The listing builds one solid part. Answer for the finished solid, in the listing's coordinates (mm). Face numbers are marked on the shaded views. A direction names the side the tool comes from. Coordinates: 2 decimals unless noted, no trailing zeros. Write each loop counter-clockwise with the first axis right and the second up, starting at its lowest first coordinate (ties: lowest second). Pieces come first, ordered by that corner, then holes.
from build123d import *

# Parameters (mm, degrees)
BASE_FLANGE1_DEPTH             = 120.65
BASE_FLANGE1_DEPTH_BACK        = 120.65
SKETCH2_W                      = 279.4
SKETCH2_H                      = 1.5875
EDGE_FLANGE1_STRIP_W           = 19.05
EDGE_FLANGE1_STRIP_H           = 1.5875
EDGE_FLANGE1_STRIP_CUT_DEPTH   = 279.4
EDGE_FLANGE1_STRIP_2_W         = 19.05
EDGE_FLANGE1_STRIP_2_H         = 1.5875
EDGE_FLANGE1_STRIP_CUT_2_DEPTH = 279.4
EDGE_FLANGE1_DEPTH             = 279.4
EDGE_FLANGE1_BEND_DEPTH        = 279.4
EDGE_FLANGE2_STRIP_W           = 16.51
EDGE_FLANGE2_STRIP_H           = 1.5875
EDGE_FLANGE2_STRIP_CUT_DEPTH   = 279.4
EDGE_FLANGE2_STRIP_2_W         = 16.51
EDGE_FLANGE2_STRIP_2_H         = 1.5875
EDGE_FLANGE2_STRIP_CUT_2_DEPTH = 279.4
EDGE_FLANGE2_DEPTH             = 279.4
EDGE_FLANGE2_BEND_DEPTH        = 279.4
FILLET1_R                      = 6.35
SKETCH18_R                     = 2.38125
CUT_EXTRUDE1_DEPTH             = 200.096804736
CUT_EXTRUDE2_REACH             = 201.097
SKETCH19_R                     = 6.35


# Sheet-metal steps are written as plain solids
with BuildPart() as part:
    # Sketch2 → Base-Flange1 (new, two sides: drawn at the far end of the back side and taken through both)
    with BuildSketch(Plane.XY.offset(-BASE_FLANGE1_DEPTH_BACK)):
        with Locations((0, -0.79375)):
            Rectangle(SKETCH2_W, SKETCH2_H)
    extrude(amount=BASE_FLANGE1_DEPTH + BASE_FLANGE1_DEPTH_BACK)

    # Edge-Flange1 strip (across the edge) → Edge-Flange1 strip cut (cut)
    with BuildSketch(Plane(origin=(139.7, -1.5875, 120.65), x_dir=(0, 0, -1), z_dir=(-1, 0, 0))):
        with Locations((-1.5875, -0.79375)):
            Rectangle(EDGE_FLANGE1_STRIP_W, EDGE_FLANGE1_STRIP_H)
    extrude(amount=EDGE_FLANGE1_STRIP_CUT_DEPTH, mode=Mode.SUBTRACT)

    # Edge-Flange1 strip 2 (across the edge) → Edge-Flange1 strip cut 2 (cut)
    with BuildSketch(Plane(origin=(-139.7, -1.5875, -120.65), x_dir=(0, 0, 1), z_dir=(1, 0, 0))):
        with Locations((-1.5875, -0.79375)):
            Rectangle(EDGE_FLANGE1_STRIP_2_W, EDGE_FLANGE1_STRIP_2_H)
    extrude(amount=EDGE_FLANGE1_STRIP_CUT_2_DEPTH, mode=Mode.SUBTRACT)

    # Edge-Flange1 section (across the edge) → Edge-Flange1 (add)
    with BuildSketch(Plane(origin=(139.7, -1.5875, 120.65), x_dir=(0, 0, -1), z_dir=(-1, 0, 0))):
        with BuildLine():
            Line((0, 6.35), (0, 73.025))
            Line((0, 73.025), (1.5875, 73.025))
            Line((1.5875, 73.025), (1.5875, 6.35))
            ThreePointArc((1.5875, 6.35), (3.447371939, 1.859871939), (7.9375, 0))
            Line((7.9375, 0), (7.9375, -1.5875))
            ThreePointArc((7.9375, -1.5875), (2.324839924, 0.737339924), (0, 6.35))
        make_face()
    extrude(amount=EDGE_FLANGE1_DEPTH)

    # Edge-Flange1 section 2 (across the edge) → Edge-Flange1 bend (add)
    with BuildSketch(Plane(origin=(-139.7, -1.5875, -120.65), x_dir=(0, 0, 1), z_dir=(1, 0, 0))):
        with BuildLine():
            Line((0, 6.35), (0, 73.025))
            Line((0, 73.025), (1.5875, 73.025))
            Line((1.5875, 73.025), (1.5875, 6.35))
            ThreePointArc((1.5875, 6.35), (3.447371939, 1.859871939), (7.9375, 0))
            Line((7.9375, 0), (7.9375, -1.5875))
            ThreePointArc((7.9375, -1.5875), (2.324839924, 0.737339924), (0, 6.35))
        make_face()
    extrude(amount=EDGE_FLANGE1_BEND_DEPTH)

    # Edge-Flange2 strip (across the edge) → Edge-Flange2 strip cut (cut)
    with BuildSketch(Plane(origin=(139.7, -74.6125, 119.0625), x_dir=(0, 1, 0), z_dir=(-1, 0, 0))):
        with Locations((-1.5875, -0.79375)):
            Rectangle(EDGE_FLANGE2_STRIP_W, EDGE_FLANGE2_STRIP_H)
    extrude(amount=EDGE_FLANGE2_STRIP_CUT_DEPTH, mode=Mode.SUBTRACT)

    # Edge-Flange2 strip 2 (across the edge) → Edge-Flange2 strip cut 2 (cut)
    with BuildSketch(Plane(origin=(-139.7, -74.6125, -119.0625), x_dir=(0, 1, 0), z_dir=(1, 0, 0))):
        with Locations((-1.5875, -0.79375)):
            Rectangle(EDGE_FLANGE2_STRIP_2_W, EDGE_FLANGE2_STRIP_2_H)
    extrude(amount=EDGE_FLANGE2_STRIP_CUT_2_DEPTH, mode=Mode.SUBTRACT)

    # Edge-Flange2 section (across the edge) → Edge-Flange2 (add)
    with BuildSketch(Plane(origin=(139.7, -74.6125, 119.0625), x_dir=(0, 1, 0), z_dir=(-1, 0, 0))):
        with BuildLine():
            Line((0, 5.08), (0, 23.8125))
            Line((0, 23.8125), (1.5875, 23.8125))
            Line((1.5875, 23.8125), (1.5875, 5.08))
            ThreePointArc((1.5875, 5.08), (3.075397552, 1.487897552), (6.6675, 0))
            Line((6.6675, 0), (6.6675, -1.5875))
            ThreePointArc((6.6675, -1.5875), (1.952865536, 0.365365536), (0, 5.08))
        make_face()
    extrude(amount=EDGE_FLANGE2_DEPTH)

    # Edge-Flange2 section 2 (across the edge) → Edge-Flange2 bend (add)
    with BuildSketch(Plane(origin=(-139.7, -74.6125, -119.0625), x_dir=(0, 1, 0), z_dir=(1, 0, 0))):
        with BuildLine():
            Line((0, 5.08), (0, 23.8125))
            Line((0, 23.8125), (1.5875, 23.8125))
            Line((1.5875, 23.8125), (1.5875, 5.08))
            ThreePointArc((1.5875, 5.08), (3.075397552, 1.487897552), (6.6675, 0))
            Line((6.6675, 0), (6.6675, -1.5875))
            ThreePointArc((6.6675, -1.5875), (1.952865536, 0.365365536), (0, 5.08))
        make_face()
    extrude(amount=EDGE_FLANGE2_BEND_DEPTH)

    # Fillet1
    fillet1_edges = [part.edges().sort_by_distance(p)[0] for p in [
        (139.7, -73.81875, 95.25),
        (-139.7, -73.81875, 95.25),
        (-139.7, -73.81875, -95.25),
        (139.7, -73.81875, -95.25),
    ]]
    fillet(fillet1_edges, radius=FILLET1_R)

    # Sketch18 → Cut-Extrude1 (cut, through all)
    with BuildSketch(Plane.XZ.offset(74.6125)):
        with Locations(Location((-107.95, 104.61625, 0), (0, 0, 270))):
            Circle(SKETCH18_R)
        with Locations(Location((-107.95, -104.61625, 0), (0, 0, 270))):
            Circle(SKETCH18_R)
        with Locations(Location((107.95, -104.61625, 0), (0, 0, 270))):
            Circle(SKETCH18_R)
        with Locations(Location((107.95, 104.61625, 0), (0, 0, 270))):
            Circle(SKETCH18_R)
    extrude(amount=-CUT_EXTRUDE1_DEPTH, mode=Mode.SUBTRACT)

    # Sketch19 → Cut-Extrude2 (cut, up to next)
    with BuildSketch(Plane(origin=(0, 0, 0), x_dir=(1, 0, 0), z_dir=(0, 1, 0)), mode=Mode.PRIVATE) as cut_extrude2_sk1:
        with Locations(Location((-107.95, -104.61625, 0), (0, 0, 180))):
            Circle(SKETCH19_R)
    cut_extrude2_tool1 = extrude(cut_extrude2_sk1.sketch, amount=-CUT_EXTRUDE2_REACH, mode=Mode.PRIVATE) & part.part
    # Sketch19 → Cut-Extrude2 (cut, up to next)
    with BuildSketch(Plane(origin=(0, 0, 0), x_dir=(1, 0, 0), z_dir=(0, 1, 0)), mode=Mode.PRIVATE) as cut_extrude2_sk2:
        with Locations(Location((107.95, -104.61625, 0), (0, 0, 180))):
            Circle(SKETCH19_R)
    cut_extrude2_tool2 = extrude(cut_extrude2_sk2.sketch, amount=-CUT_EXTRUDE2_REACH, mode=Mode.PRIVATE) & part.part
    # Sketch19 → Cut-Extrude2 (cut, up to next)
    with BuildSketch(Plane(origin=(0, 0, 0), x_dir=(1, 0, 0), z_dir=(0, 1, 0)), mode=Mode.PRIVATE) as cut_extrude2_sk3:
        with Locations(Location((107.95, 104.61625, 0), (0, 0, 180))):
            Circle(SKETCH19_R)
    cut_extrude2_tool3 = extrude(cut_extrude2_sk3.sketch, amount=-CUT_EXTRUDE2_REACH, mode=Mode.PRIVATE) & part.part
    # Sketch19 → Cut-Extrude2 (cut, up to next)
    with BuildSketch(Plane(origin=(0, 0, 0), x_dir=(1, 0, 0), z_dir=(0, 1, 0)), mode=Mode.PRIVATE) as cut_extrude2_sk4:
        with Locations(Location((-107.95, 104.61625, 0), (0, 0, 180))):
            Circle(SKETCH19_R)
    cut_extrude2_tool4 = extrude(cut_extrude2_sk4.sketch, amount=-CUT_EXTRUDE2_REACH, mode=Mode.PRIVATE) & part.part
    add(cut_extrude2_tool1.solids().sort_by_distance((-107.95, 0, 104.61625))[0], mode=Mode.SUBTRACT)
    add(cut_extrude2_tool2.solids().sort_by_distance((107.95, 0, 104.61625))[0], mode=Mode.SUBTRACT)
    add(cut_extrude2_tool3.solids().sort_by_distance((107.95, 0, -104.61625))[0], mode=Mode.SUBTRACT)
    add(cut_extrude2_tool4.solids().sort_by_distance((-107.95, 0, -104.61625))[0], mode=Mode.SUBTRACT)


solid = part.part
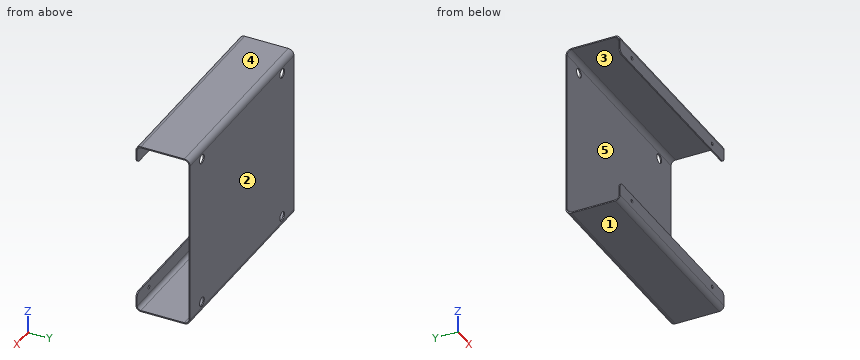
Q1. Determine the mould class of the marked faces 1, 2 and 3 for opening direction Y: released by +Y, released by -Y, zero draft, split by the parting line, or undercut.
Answers below:
face 1: zero draft
face 2: released by +Y
face 3: undercut
Q2. The part is cut by section A-A, the plane y = -14.5. Write down the section's boundary in (x, z).
Answers below:
outline: (-139.7, -120.65) - (139.7, -120.65) - (139.7, -119.06) - (-139.7, -119.06) - close; (-139.7, 119.06) - (139.7, 119.06) - (139.7, 120.65) - (-139.7, 120.65) - close
Q3. The part is cut by section C-C, the plane z = 84. Write down the section's boundary in (x, y), then the cut area to 3 significant figures.
Answers below:
outline: (-139.7, -1.59) - (139.7, -1.59) - (139.7, 0) - (-139.7, 0) - close
area: 444 mm2
Q4. Find the intervals of material crossed by probe 1 along Z at (x, y) = (83, -8.5); probe 2 along Y at (x, z) = (110.5, -96) (1 decimal), in increasing order.
Answers below:
probe 1: z = -120.65 to -119.06, 119.06 to 120.65
probe 2: y = -74.6 to -73, -1.6 to 0
Q5. Which of the six approach directions +Z, -Z, +X, -X, +Y, -Y give full straight-line access (tool end or side, diameter ignored) to the marked faces 4 and 5?
Answers below:
face 4: +Z, +X, -X, +Y, -Y
face 5: +X, -X
Q6. Given pin 1 (11.5 mm diameter, centred on x = -107.95, z = -104.62, fed in from -Y); pin 2 (0.5 mm diameter, centred on x = 3, y = -74, fed in from +Z); pin 3 (3 mm diameter, centred on x = -100, z = -69, fed in from -Y); pin 4 (1.7 mm diameter, centred on x = -14, y = -74, fed in from -Z), each flat-ended and moving along its own axis, determine where each tip first touches the part or whether it passes through.
Answers below:
pin 1: stops at y = -74.61
pin 2: stops at z = 117.26
pin 3: stops at y = -1.59
pin 4: stops at z = -118.15
